Verification items for the finished model (mm, model axes). A direction names the side the tool comes from. Give positions to 0.01 mm unless a question says otherwise; leave off trailing zeros. Write each loop counter-clockwise with the first axis right and the second up, starting at its lowest first coordinate (ties: lowest second). Pieces come first, ordered by that corner, then holes. Notation, with made-up numbers: (38.5, 79) - (83.5, 79) arc R19 cw to (83.5, 99) - close; hole circle Ø10 at (34.25, 79.25). An arc over 180 degrees is marked (long way). Answer as a JSON object with one key per item and string values. Group by question number.
Item 1: Sectioned sample at B-B, the plane z = 0. Record the boundary of the cut face in (x, y) (1 decimal), and give its area (3 significant figures).
Item 2: Scan lines: line 1 along X through (y, z) = (10.75, -3.75); line 2 along X through (y, z) = (14.25, 2); line 3 along Z through (x, y) = (-28, 13). Record each from-to range of solid material in increasing order. Write a range as [from, to].
Item 3: Sectioned sample at A-A, the plane y = 11. Count the separate pieces of the cut face and the enclosed holes in it, and give its area (3 significant figures).
Item 4: Go/stop test with flat-tipped pins: pin 1 (9.5 mm diameter, centred on x = 31.5, z = 4.5, fed in from +Y); pin 2 (6 mm diameter, centred on x = 1.5, z = -9, fed in from -Y); pin 3 (10 mm diameter, centred on x = -9, y = 5, fed in from -Z); pin 4 (12 mm diameter, centred on y = 17, z = 6.5, fed in from +X). Record where each tip stops, or that it passes through.
Item 5: Draft check along X on faces 6 (the face through (20.878, 15.834, -0.178)), 7 (the face through (-29, 0, -3)), 8 (the face through (0, 20, 0)). Enter one of: +X half, -X half, draft (parallel to the pull), parting line (faces both ways), or undercut.
Item 6: Sectioned sample at D-D, the plane x = 0. Record the boundary of the cut face in (y, z), and give its area (3 significant figures).
Item 7: Tool access check on faces 1 (the face through (-42.54, 7.51, -0.28)), 2 (the face through (37.215, 15.24, -2.644)), 3 (the face through (-34.444, 4.696, 0.14)), 4 (the face through (34, 9.525, 2)), 5 (the face through (-37.5, 15.24, -2.6)). Record the directions out of +Z, -Z, +X, -X, +Y, -Y that give a thin tool (end or side, any length) a straight path to the whole face; none if there is none.
Item 8: Sectioned sample at C-C, the plane z = 10.5. Record the boundary of the cut face in (x, y).
```python
from build123d import *

# Parameters (mm, degrees)
BOSS_EXTRUDE1_DEPTH = 12.7
FILLET1_R           = 7.62
FILLET2_R           = 7.62
SKETCH2_R           = 3.175
CUT_EXTRUDE1_DEPTH  = 9.525
SKETCH3_R           = 6.35
CUT_EXTRUDE2_DEPTH  = 5.715
SKETCH4_OUTSIDE_W   = 105.562
SKETCH4_OUTSIDE_H   = 45.872
CUT_EXTRUDE3_DEPTH  = 26.4


with BuildPart() as part:
    # Sketch1 → Boss-Extrude1 (new body, symmetric)
    with BuildSketch(Plane.XY):
        with BuildLine():
            Line((-42.545, 0), (-42.545, 15.24))
            Line((-42.545, 15.24), (-20.32, 15.24))
            ThreePointArc((-20.32, 15.24), (0, 25.4), (20.32, 15.24))
            Line((20.32, 15.24), (42.545, 15.24))
            Line((42.545, 15.24), (42.545, 0))
            Line((42.545, 0), (20, 0))
            ThreePointArc((20, 0), (0, 20), (-20, 0))
            Line((-20, 0), (-42.545, 0))
        make_face()
    extrude(amount=BOSS_EXTRUDE1_DEPTH, both=True)

    # Fillet1
    fillet1_edges = [part.edges().sort_by_distance(p)[0] for p in [
        (20.32, 15.24, 0),
    ]]
    fillet(fillet1_edges, radius=FILLET1_R)

    # Fillet2
    fillet2_edges = [part.edges().sort_by_distance(p)[0] for p in [
        (-20.32, 15.24, 0),
    ]]
    fillet(fillet2_edges, radius=FILLET2_R)

    # Sketch2 → Cut-Extrude1 (cut)
    with BuildSketch(Plane.XZ):
        with Locations((-31.2725, 0)):
            Circle(SKETCH2_R)
    cut_extrude1 = extrude(amount=-CUT_EXTRUDE1_DEPTH, mode=Mode.SUBTRACT)

    # Sketch3 → Cut-Extrude2 (cut)
    with BuildSketch(Plane.XZ.offset(-9.525)):
        with Locations((-31.2725, 0)):
            Circle(SKETCH3_R)
    cut_extrude2 = extrude(amount=-CUT_EXTRUDE2_DEPTH, mode=Mode.SUBTRACT)

    # Mirror1: Cut-Extrude1, Cut-Extrude2 across plane
    add(cut_extrude1.mirror(Plane(origin=(0, 0, 0), x_dir=(0, 0, 1), z_dir=(1, 0, 0))), mode=Mode.SUBTRACT)
    add(cut_extrude2.mirror(Plane(origin=(0, 0, 0), x_dir=(0, 0, 1), z_dir=(1, 0, 0))), mode=Mode.SUBTRACT)

    # Sketch4 outside → Cut-Extrude3 (cut, through all)
    with BuildSketch(Plane(origin=(0, 0, 0), x_dir=(1, 0, 0), z_dir=(0, 1, 0))):
        Rectangle(SKETCH4_OUTSIDE_W, SKETCH4_OUTSIDE_H)
        with BuildLine():
            Line((-29.845, -12.7), (29.845, -12.7))
            ThreePointArc((29.845, -12.7), (42.545, 0), (29.845, 12.7))
            Line((29.845, 12.7), (-29.845, 12.7))
            ThreePointArc((-29.845, 12.7), (-42.545, 0), (-29.845, -12.7))
        make_face(mode=Mode.SUBTRACT)
    extrude(amount=CUT_EXTRUDE3_DEPTH, mode=Mode.SUBTRACT)


solid = part.part
```
Geometry check:
{
 "1": {"outline": "(-42.5, 0) - (-34.4, 0) - (-34.4, 9.5) - (-37.6, 9.5) - (-37.6, 15.2) - (-42.5, 15.2) - close; (-28.1, 0) - (-20, 0) arc R20 cw to (20, 0) - (28.1, 0) - (28.1, 9.5) - (24.9, 9.5) - (24.9, 15.2) - (23.8, 15.2) arc R7.6 cw to (18.3, 17.6) arc R25.4 ccw to (-18.3, 17.6) arc R7.6 cw to (-23.8, 15.2) - (-24.9, 15.2) - (-24.9, 9.5) - (-28.1, 9.5) - close; (34.4, 0) - (42.5, 0) - (42.5, 15.2) - (37.6, 15.2) - (37.6, 9.5) - (34.4, 9.5) - close", "area": "694 mm^2"},
 "2": {"line 1": "[-41.98, -36.4], [-26.15, -16.87], [16.87, 26.15], [36.4, 41.98]", "line 2": "[-42.39, -37.3], [-25.25, -14.03], [14.03, 25.25], [37.3, 42.39]", "line 3": "[-12.7, -5.44], [5.44, 12.7]"},
 "3": {"separate pieces": "2", "enclosed holes": "2", "area": "921 mm^2"},
 "4": {"pin 1": "y = 15.24", "pin 2": "y = 19.49", "pin 3": "through", "pin 4": "x = 42.52"},
 "5": {"face 6": "+X half", "face 7": "draft", "face 8": "undercut"},
 "6": {"outline": "(20, -12.7) - (25.4, -12.7) - (25.4, 12.7) - (20, 12.7) - close", "area": "137 mm^2"},
 "7": {"face 1": "-X, +Y, -Y", "face 2": "+Z, -Z, +X, +Y", "face 3": "+Y, -Y", "face 4": "+Y", "face 5": "+Z, -Z, -X, +Y"},
 "8": {"outline": "(-36.99, 0) - (-20, 0) arc R20 cw to (20, 0) - (36.99, 0) - (36.99, 15.24) - (23.83, 15.24) arc R7.62 cw to (18.33, 17.58) arc R25.4 ccw to (-18.33, 17.58) arc R7.62 cw to (-23.83, 15.24) - (-36.99, 15.24) - close"}
}
